Design review of the part built by this model. Coordinates are the model's own, in mm. A direction names the side the tool comes from. Coordinates: 2 decimals unless noted, no trailing zeros.
Q1. Take a section at A-A, the plane y = -17. State how many separate pieces and enclosed holes the cut face has, plus the area to 3 significant figures.
Q2. The part is to be moulded in two halves that separate along Y. For faces 3 (the cylindrical face through (-21.95, -30.81, 28.25)), 4 (the flat face through (-22.2, -37, -12)), 5 (the flat face through (1.97, -5.22, 2.96)), say which applies: released by +Y, released by -Y, zero draft, split by the parting line, or undercut.
Q3. For pin 1 Ø1 at (y, z) = (16.5, -10.5) entering from +X; pin 2 Ø1.2 at (x, y) = (3, -1.5) entering from -Z; pin 3 Ø3 at (x, z) = (-9, 0) entering from -Y; pin 4 Ø4 at (y, z) = (2.5, -22.5) entering from +X, all flat-tipped, find the tip position at first contact; note any pin that passes through.
Q4. For faces 1 (the flat face through (0, 5, -4)), 2 (the cylindrical face through (15, 12, 0)), list the 3-axis set-ups (+Z, -Z, +X, -X, +Y, -Y) from which the entire face can be reached by the end or side of a thin tool; tool diameter is ignored.
Q5. For L1, parallel to Y at x = 8, z = 10; L2, parallel to Y at x = 13, z = 32.5; L3, parallel to Y at x = -17, z = 23.5, list the stretches that pass through material, from the lowest coordinate up.
from build123d import *

# Parameters (mm, degrees)
CUT_EXTRUDE1_REACH = 32.2
SKETCH3_R          = 2.15
CUT_EXTRUDE2_REACH = 45.668
CUT_EXTRUDE3_DEPTH = 4


with BuildPart() as part:
    # Sketch2 → Revolve1 (revolve)
    with BuildSketch(Plane.XY):
        with BuildLine():
            Line((0, 0), (0, 9.871675482))
            Line((0, 9.871675482), (16.488909248, 13.365088458))
            Line((16.488909248, 13.365088458), (13.847020393, 35))
            Line((13.847020393, 35), (-22.2, 38.5))
            Line((-22.2, 38.5), (-22.2, 41.8))
            Line((-22.2, 41.8), (-21.7, 41.8))
            add(Edge.make_bspline(
                [(-21.7, 41.8), (-21.533718516, 55.260750985), (-4.008905518, 53.174245615), (23.517269043, 55.137002211), (21.925848048, 36.077457734), (21.468315468, 30)],
                knots=[0, 0, 0, 0, 0.416041418, 0.696055302, 1, 1, 1, 1], degree=3))
            Line((21.468315468, 30), (21.468315468, 26))
            Line((21.468315468, 26), (17.968315468, 26))
            Line((17.968315468, 26), (19.8, 11))
            Line((19.8, 11), (8, 8.5))
            Line((8, 8.5), (8, 0))
            Line((8, 0), (0, 0))
        make_face()
    revolve(axis=Axis((-63.183775164, 0, 0), (1, 0, 0)))

    # Sketch3 → Cut-Extrude1 (cut, up to next)
    with BuildSketch(Plane(origin=(8, 0, 0), x_dir=(0, 0, -1), z_dir=(1, 0, 0)), mode=Mode.PRIVATE) as cut_extrude1_sk1:
        Circle(SKETCH3_R)
    cut_extrude1_tool1 = extrude(cut_extrude1_sk1.sketch, amount=-CUT_EXTRUDE1_REACH, mode=Mode.PRIVATE) & part.part
    add(cut_extrude1_tool1.solids().sort_by_distance((8, 0, 0))[0], mode=Mode.SUBTRACT)

    # Sketch4 → Cut-Extrude2 (cut, up to next)
    with BuildSketch(Plane(origin=(21.468315468, 0, 0), x_dir=(0, 0, -1), z_dir=(1, 0, 0)), mode=Mode.PRIVATE) as cut_extrude2_sk1:
        with BuildLine():
            Line((-8.51429142, 20.225424859), (8.51429142, 20.225424859))
            Line((8.51429142, 20.225424859), (10.352654493, 22.755714556))
            ThreePointArc((10.352654493, 22.755714556), (0, 25), (-10.352654493, 22.755714556))
            Line((-10.352654493, 22.755714556), (-8.51429142, 20.225424859))
        make_face()
    cut_extrude2_tool1 = extrude(cut_extrude2_sk1.sketch, amount=-CUT_EXTRUDE2_REACH, mode=Mode.PRIVATE) & part.part
    add(cut_extrude2_tool1.solids().sort_by_distance((21.468315, 22.372787, 0))[0], mode=Mode.SUBTRACT)
    # Sketch4 → Cut-Extrude2 (cut, up to next)
    with BuildSketch(Plane(origin=(21.468315468, 0, 0), x_dir=(0, 0, -1), z_dir=(1, 0, 0)), mode=Mode.PRIVATE) as cut_extrude2_sk2:
        with BuildLine():
            Line((-8.51429142, 20.225424859), (-2.366895131, 11.764259749))
            ThreePointArc((-2.366895131, 11.764259749), (0, 12), (2.366895131, 11.764259749))
            Line((2.366895131, 11.764259749), (8.51429142, 20.225424859))
            Line((8.51429142, 20.225424859), (-8.51429142, 20.225424859))
        make_face()
    cut_extrude2_tool2 = extrude(cut_extrude2_sk2.sketch, amount=-CUT_EXTRUDE2_REACH, mode=Mode.PRIVATE) & part.part
    add(cut_extrude2_tool2.solids().sort_by_distance((21.468315, 16.831807, 0))[0], mode=Mode.SUBTRACT)
    # Sketch4 → Cut-Extrude2 (cut, up to next)
    with BuildSketch(Plane(origin=(21.468315468, 0, 0), x_dir=(0, 0, -1), z_dir=(1, 0, 0)), mode=Mode.PRIVATE) as cut_extrude2_sk3:
        with BuildLine():
            Line((16.604461364, 14.347572336), (21.866582851, -1.847572336))
            Line((21.866582851, -1.847572336), (24.841116787, -2.814056999))
            ThreePointArc((24.841116787, -2.814056999), (24.960247592, -1.409269374), (25, 0))
            ThreePointArc((25, 0), (23.303117934, 9.053435511), (18.442824436, 16.877862033))
            Line((18.442824436, 16.877862033), (16.604461364, 14.347572336))
        make_face()
    cut_extrude2_tool3 = extrude(cut_extrude2_sk3.sketch, amount=-CUT_EXTRUDE2_REACH, mode=Mode.PRIVATE) & part.part
    add(cut_extrude2_tool3.solids().sort_by_distance((21.468315, 6.913571, -21.277785))[0], mode=Mode.SUBTRACT)
    # Sketch4 → Cut-Extrude2 (cut, up to next)
    with BuildSketch(Plane(origin=(21.468315468, 0, 0), x_dir=(0, 0, -1), z_dir=(1, 0, 0)), mode=Mode.PRIVATE) as cut_extrude2_sk4:
        with BuildLine():
            Line((11.919886713, 1.384305151), (21.866582851, -1.847572336))
            Line((21.866582851, -1.847572336), (16.604461364, 14.347572336))
            Line((16.604461364, 14.347572336), (10.457065074, 5.886407226))
            ThreePointArc((10.457065074, 5.886407226), (11.412678196, 3.708203932), (11.919886713, 1.384305151))
        make_face()
    cut_extrude2_tool4 = extrude(cut_extrude2_sk4.sketch, amount=-CUT_EXTRUDE2_REACH, mode=Mode.PRIVATE) & part.part
    add(cut_extrude2_tool4.solids().sort_by_distance((21.468315, 5.201314, -16.007999))[0], mode=Mode.SUBTRACT)
    # Sketch4 → Cut-Extrude2 (cut, up to next)
    with BuildSketch(Plane(origin=(21.468315468, 0, 0), x_dir=(0, 0, -1), z_dir=(1, 0, 0)), mode=Mode.PRIVATE) as cut_extrude2_sk5:
        with BuildLine():
            Line((18.776412907, -11.358137499), (5, -21.36728736))
            Line((5, -21.36728736), (5, -24.494897428))
            ThreePointArc((5, -24.494897428), (14.694631307, -20.225424859), (21.750946843, -12.324622162))
            Line((21.750946843, -12.324622162), (18.776412907, -11.358137499))
        make_face()
    cut_extrude2_tool5 = extrude(cut_extrude2_sk5.sketch, amount=-CUT_EXTRUDE2_REACH, mode=Mode.PRIVATE) & part.part
    add(cut_extrude2_tool5.solids().sort_by_distance((21.468315, -18.099965, -13.150394))[0], mode=Mode.SUBTRACT)
    # Sketch4 → Cut-Extrude2 (cut, up to next)
    with BuildSketch(Plane(origin=(21.468315468, 0, 0), x_dir=(0, 0, -1), z_dir=(1, 0, 0)), mode=Mode.PRIVATE) as cut_extrude2_sk6:
        with BuildLine():
            Line((5, -10.908712115), (5, -21.36728736))
            Line((5, -21.36728736), (18.776412907, -11.358137499))
            Line((18.776412907, -11.358137499), (8.829716769, -8.126260012))
            ThreePointArc((8.829716769, -8.126260012), (7.053423028, -9.708203932), (5, -10.908712115))
        make_face()
    cut_extrude2_tool6 = extrude(cut_extrude2_sk6.sketch, amount=-CUT_EXTRUDE2_REACH, mode=Mode.PRIVATE) & part.part
    add(cut_extrude2_tool6.solids().sort_by_distance((21.468315, -13.617218, -9.893488))[0], mode=Mode.SUBTRACT)
    # Sketch4 → Cut-Extrude2 (cut, up to next)
    with BuildSketch(Plane(origin=(21.468315468, 0, 0), x_dir=(0, 0, -1), z_dir=(1, 0, 0)), mode=Mode.PRIVATE) as cut_extrude2_sk7:
        with BuildLine():
            Line((-5, -24.494897428), (-5, -21.36728736))
            Line((-5, -21.36728736), (-18.776412907, -11.358137499))
            Line((-18.776412907, -11.358137499), (-21.750946843, -12.324622162))
            ThreePointArc((-21.750946843, -12.324622162), (-14.694631307, -20.225424859), (-5, -24.494897428))
        make_face()
    cut_extrude2_tool7 = extrude(cut_extrude2_sk7.sketch, amount=-CUT_EXTRUDE2_REACH, mode=Mode.PRIVATE) & part.part
    add(cut_extrude2_tool7.solids().sort_by_distance((21.468315, -18.099965, 13.150394))[0], mode=Mode.SUBTRACT)
    # Sketch4 → Cut-Extrude2 (cut, up to next)
    with BuildSketch(Plane(origin=(21.468315468, 0, 0), x_dir=(0, 0, -1), z_dir=(1, 0, 0)), mode=Mode.PRIVATE) as cut_extrude2_sk8:
        with BuildLine():
            Line((-18.776412907, -11.358137499), (-5, -21.36728736))
            Line((-5, -21.36728736), (-5, -10.908712115))
            ThreePointArc((-5, -10.908712115), (-7.053423028, -9.708203932), (-8.829716769, -8.126260012))
            Line((-8.829716769, -8.126260012), (-18.776412907, -11.358137499))
        make_face()
    cut_extrude2_tool8 = extrude(cut_extrude2_sk8.sketch, amount=-CUT_EXTRUDE2_REACH, mode=Mode.PRIVATE) & part.part
    add(cut_extrude2_tool8.solids().sort_by_distance((21.468315, -13.617218, 9.893488))[0], mode=Mode.SUBTRACT)
    # Sketch4 → Cut-Extrude2 (cut, up to next)
    with BuildSketch(Plane(origin=(21.468315468, 0, 0), x_dir=(0, 0, -1), z_dir=(1, 0, 0)), mode=Mode.PRIVATE) as cut_extrude2_sk9:
        with BuildLine():
            Line((-24.841116787, -2.814056999), (-21.866582851, -1.847572336))
            Line((-21.866582851, -1.847572336), (-16.604461364, 14.347572336))
            Line((-16.604461364, 14.347572336), (-18.442824436, 16.877862033))
            ThreePointArc((-18.442824436, 16.877862033), (-23.776412907, 7.725424859), (-24.841116787, -2.814056999))
        make_face()
    cut_extrude2_tool9 = extrude(cut_extrude2_sk9.sketch, amount=-CUT_EXTRUDE2_REACH, mode=Mode.PRIVATE) & part.part
    add(cut_extrude2_tool9.solids().sort_by_distance((21.468315, 6.913571, 21.277785))[0], mode=Mode.SUBTRACT)
    # Sketch4 → Cut-Extrude2 (cut, up to next)
    with BuildSketch(Plane(origin=(21.468315468, 0, 0), x_dir=(0, 0, -1), z_dir=(1, 0, 0)), mode=Mode.PRIVATE) as cut_extrude2_sk10:
        with BuildLine():
            Line((-16.604461364, 14.347572336), (-21.866582851, -1.847572336))
            Line((-21.866582851, -1.847572336), (-11.919886713, 1.384305151))
            ThreePointArc((-11.919886713, 1.384305151), (-11.412678196, 3.708203932), (-10.457065074, 5.886407226))
            Line((-10.457065074, 5.886407226), (-16.604461364, 14.347572336))
        make_face()
    cut_extrude2_tool10 = extrude(cut_extrude2_sk10.sketch, amount=-CUT_EXTRUDE2_REACH, mode=Mode.PRIVATE) & part.part
    add(cut_extrude2_tool10.solids().sort_by_distance((21.468315, 5.201314, 16.007999))[0], mode=Mode.SUBTRACT)

    # Sketch5 → Cut-Extrude3 (cut)
    with BuildSketch(Plane.ZY):
        Polygon((0, -6.92820323), (6, -3.464101615), (6, 3.464101615), (0, 6.92820323), (-6, 3.464101615), (-6, -3.464101615), align=None)
    extrude(amount=-CUT_EXTRUDE3_DEPTH, mode=Mode.SUBTRACT)


solid = part.part
Responses:
1. separate pieces: 3
1. enclosed holes: 0
1. area: 1,730 mm2
2. face 3: split by the parting line
2. face 4: zero draft
2. face 5: undercut
3. pin 1: stops at x = 18.82
3. pin 2: stops at z = -54.01
3. pin 3: stops at y = -54.01
3. pin 4: passes through
4. face 1: -X
4. face 2: +X, -X
5. L1: y = -53.03 to -34.13, -5.81 to 5.81, 34.13 to 53.03
5. L2: y = -42.39 to -13.21, 13.21 to 42.39
5. L3: y = -46.41 to -29.86, 29.86 to 46.41
